Here's how the part is built. I have some questions about the finished solid (model axes, mm). Coordinates: 2 decimals unless noted, no trailing zeros. Order: outer loops, then holes, each group sorted by start corner. A loop starts at its lowest first (then second) coordinate and runs counter-clockwise, first axis right, second up. Notation, with made-up numbers: (-36.5, 44.5) - (0.5, 44.5) arc R21 cw to (0.5, 76.5) - close; hole circle Ø8 at (28, -16). An arc over 180 degrees is marked (long way). Answer as CSV lines item,"result". Start each with the question number.
Q1. Suppose I cut it at D-D (z = 165). Please give me the cut outline in (x, y).
Q2. I need wall thicknesses on line 1 (X direction, y = 1, z = 45); line 2 (Y direction, x = 22, z = 186); line 3 (X direction, y = 14.25, z = 37). Which ranges of each line are inside material? Lowest first, please.
Q3. Suppose I cut it at B-B (x = 6.25). Please give me the cut outline in (y, z).
Q4. For pin 1 Ø2 at (y, z) = (4, 196) entering from +X; pin 2 Ø3 at (y, z) = (11.5, 140) entering from +X; pin 3 Ø1.5 at (y, z) = (19, 99) entering from +X, each with a flat end and sliding along its axis, tell me the tip position at first contact or that it passes through.
Q5. Suppose I cut it at C-C (y = 19.5). Please give me the cut outline in (x, z).
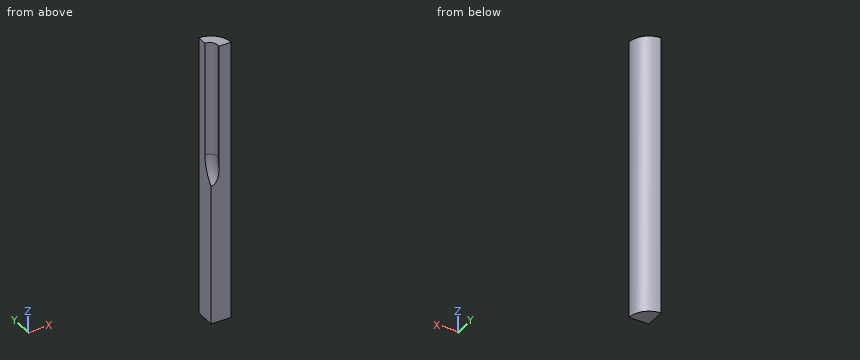
from build123d import *

# Parameters (mm, degrees)
BOSS_EXTRUDE1_DEPTH = 350
CUT_EXTRUDE1_DEPTH  = 10
FILLET1_R           = 10


with BuildPart() as part:
    # Sketch1 → Boss-Extrude1 (new body)
    with BuildSketch(Plane.XY):
        with BuildLine():
            Line((0, 0), (0, 25))
            ThreePointArc((0, 25), (17.67766953, 17.67766953), (25, 0))
            Line((25, 0), (0, 0))
        make_face()
    extrude(amount=BOSS_EXTRUDE1_DEPTH)

    # Sketch2 → Cut-Extrude1 (cut)
    with BuildSketch(Plane.ZY):
        with BuildLine():
            Line((350, 0), (350, 12.5))
            Line((350, 12.5), (208.071891388, 12.5))
            ThreePointArc((208.071891388, 12.5), (190.394221859, 9.270717335), (175, 0))
            Line((175, 0), (350, 0))
        make_face()
    extrude(amount=-CUT_EXTRUDE1_DEPTH, mode=Mode.SUBTRACT)

    # Fillet1
    fillet1_edges = [part.edges().sort_by_distance(p)[0] for p in [
        (10, 12.5, 279.035945694),
        (10, 9.270717335, 190.394221859),
    ]]
    fillet(fillet1_edges, radius=FILLET1_R - 0.0001)  # a hair under: the kernel refuses the full size


solid = part.part
Here are the results:
1,outline,"(0, 0) - (25, 0) arc R25 ccw to (0, 25) - close"
2,line 1,"x = 0 to 24.98"
2,line 2,"y = 0 to 11.87"
2,line 3,"x = 0 to 20.54"
3,outline,"(0, 0) - (24.21, 0) - (24.21, 350) - (10.31, 350) - (10.31, 208.07) arc R47.81 cw to (0, 178.42) - close"
4,pin 1,"stops at x = 24.82"
4,pin 2,"stops at x = 22.91"
4,pin 3,"stops at x = 17.09"
5,outline,"(0, 0) - (15.64, 0) - (15.64, 350) - (0, 350) - close"
